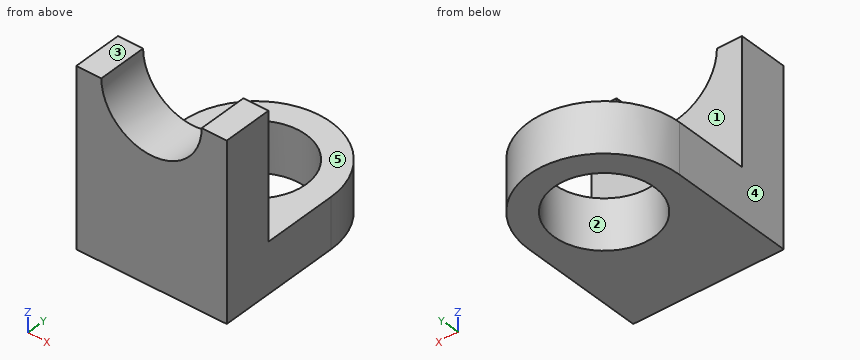
Autodesk Inventor part; units mm, degrees
ref_plane "YZ Plane" through (0, 0, 0) normal (1, 0, 0) x (0, 1, 0)
ref_plane "XZ Plane" through (0, 0, 0) normal (0, 1, 0) x (-1, 0, 0)
ref_plane "XY Plane" through (0, 0, 0) normal (0, 0, 1) x (1, 0, 0)
sketch "Sketch1" plane through (0, 0, 0) normal (0, 1, 0) x (-1, 0, 0)
  line L0 (15, 17.5) -> (-15, 17.5)
  line L1 (-15, 17.5) -> (-15, -17.5)
  line L2 (-15, -17.5) -> (15, -17.5)
  line L3 (15, -17.5) -> (15, 17.5)
  line L4 (15, 17.5) -> (-15, -17.5) construction
  line L5 (-15, 17.5) -> (15, -17.5) construction
  arc A0 (-10, 17.5) -> (10, 17.5) centre (0, 17.5) ccw
  point P0 (0, 0)
  dimension "d0" = 30
  dimension "d1" = 35
  dimension "d2" = 20
extrude "Extrusion1" add sketch "Sketch1" along normal blind 10 contours L3 L2 L1 L0 A0
sketch "Sketch2" plane through (0, 10, 0) normal (0, 1, 0) x (1, 0, 0)
  line L0 (15, 17.5) -> (-15, 17.5)
  line L1 (15, 17.5) -> (-15, 17.5)
  line L2 (-15, 17.5) -> (-15, 7.5)
  line L3 (-15, 7.5) -> (15, 7.5)
  line L4 (15, 7.5) -> (15, 17.5)
  point P0 (0, 0)
  dimension "d5" = 30
  dimension "d6" = 10
extrude "Extrusion2" add sketch "Sketch2" along normal blind 15
sketch "Sketch3" plane through (-15, 10, -7.5) normal (0, 0, 1) x (1, 0, 0)
  line L0 (0, 15) -> (30, 15)
  arc A0 (30, 15) -> (0, 15) centre (15, 15) ccw
  point P0 (15, -10)
extrude "Extrusion3" add sketch "Sketch3" against normal blind 10
sketch "Sketch4" plane through (-15, 10, -7.5) normal (0, 0, 1) x (1, 0, 0)
  arc A0 (30, 15) -> (0, 15) centre (15, 15) ccw
  circle A1 centre (15, 15) radius 10
  point P0 (15, -10)
  dimension "d12" = 20
extrude "Extrusion4" cut sketch "Sketch4" against normal blind 10
properties part number "atividade"
The listing builds one solid part. Answer for the finished solid, in the listing's coordinates (mm). Face numbers are marked on the shaded views. A direction names the side the tool comes from. Coordinates: 2 decimals unless noted, no trailing zeros. Loops run counter-clockwise (first coordinate to the right, second up) from the corner with the lowest first, then second, coordinate; pieces in that order, holes last. Notation, with made-up numbers: (80, 70.5) -> (133, 70.5) arc R16 cw to (133, 97.5) -> close; hole circle Ø7 at (18, 17.25). An arc over 180 degrees is marked (long way). Answer in a Markdown table with one row per item. Add a question column.
1. Determine the mould class of the marked faces 1, 2 and 3 for opening direction Y: +Y half, -Y half, draft (parallel to the pull), parting line (faces both ways), or undercut.
2. For the marked faces 4 and 5, determine the directions among +Z, -Z, +X, -X, +Y, -Y from which every point of the face is accessible in a straight line to the end or side of a thin tool.
3. Consider line 1 (Y direction, x = 0, z = -9.5); line 2 (Y direction, x = -10.25, z = 7.5); line 3 (Z direction, x = -4, y = 14.5). Determine where each line is inside the solid, lowest interval first. Write a range as [from, to].
4. The part is cut by section A-A, the plane x = 0. Write down the section's boundary in (y, z).
5. Flat-ended cylindrical pins translate along their axes: P1, Ø10, axis at x = 0.5, z = 0, coming from the +Y side; P2, Ø6, axis at x = 3, z = 12.5, coming from the +Y side; P3, Ø15, axis at x = -3, y = 26, coming from the +Z side. Find the tip coordinate at first contact, or state that the pin passes through.
6. The part is cut by section B-B, the plane y = 24. Write down the section's boundary in (x, z).
7. The part is cut by section C-C, the plane z = -13.5. Write down the section's boundary in (x, y), then the cut area to 3 significant figures.
8. The part is cut by section D-D, the plane z = 13. Write down the section's boundary in (x, y).
Answer below:
| question | item | result |
|---|---|---|
| 1 | face 1 | +Y half |
| 1 | face 2 | undercut |
| 1 | face 3 | draft |
| 2 | face 4 | +Z, -Z, -X, +Y, -Y |
| 2 | face 5 | +Z, +X, -X, +Y |
| 3 | line 1 | [0, 15], [35, 40] |
| 3 | line 2 | [0, 10] |
| 3 | line 3 | [-17.5, -7.5] |
| 4 | outline | (0, -17.5) -> (15, -17.5) -> (15, -7.5) -> (10, -7.5) -> (10, 7.5) -> (0, 7.5) -> close; (35, -17.5) -> (40, -17.5) -> (40, -7.5) -> (35, -7.5) -> close |
| 5 | P1 | y = 10 |
| 5 | P2 | through |
| 5 | P3 | z = -7.5 |
| 6 | outline | (-15, -17.5) -> (-9.95, -17.5) -> (-9.95, -7.5) -> (-15, -7.5) -> close; (9.95, -17.5) -> (15, -17.5) -> (15, -7.5) -> (9.95, -7.5) -> close |
| 7 | outline | (-15, 0) -> (15, 0) -> (15, 25) arc R15 ccw to (-15, 25) -> close; hole circle Ø20 at (0, 25) |
| 7 | area | 789 mm2 |
| 8 | outline | (-15, 0) -> (-8.93, 0) -> (-8.93, 10) -> (-15, 10) -> close; (8.93, 0) -> (15, 0) -> (15, 10) -> (8.93, 10) -> close |
